```python
from build123d import *

# Parameters (mm, degrees)
F1_DEPTH = 25.4


with BuildPart() as f1:
    # F0 (on Front) → F1 (new body)
    with BuildSketch(Plane.XZ):
        with BuildLine():
            Line((69.85, 31.75), (-69.85, 31.75))
            ThreePointArc((-69.85, 31.75), (-92.30064, 22.45064), (-101.6, 0))
            ThreePointArc((-101.6, 0), (-92.30064, -22.45064), (-69.85, -31.75))
            Line((-69.85, -31.75), (69.85, -31.75))
            ThreePointArc((69.85, -31.75), (92.30064, -22.45064), (101.6, 0))
            ThreePointArc((101.6, 0), (92.30064, 22.45064), (69.85, 31.75))
        make_face()
        with BuildLine():
            Line((-69.85, 25.4), (69.85, 25.4))
            ThreePointArc((69.85, 25.4), (87.810512, 17.960512), (95.25, 0))
            ThreePointArc((95.25, 0), (87.810512, -17.960512), (69.85, -25.4))
            Line((69.85, -25.4), (-69.85, -25.4))
            ThreePointArc((-69.85, -25.4), (-87.810512, -17.960512), (-95.25, 0))
            ThreePointArc((-95.25, 0), (-87.810512, 17.960512), (-69.85, 25.4))
        make_face(mode=Mode.SUBTRACT)
    extrude(amount=F1_DEPTH)


solid = f1.part
```
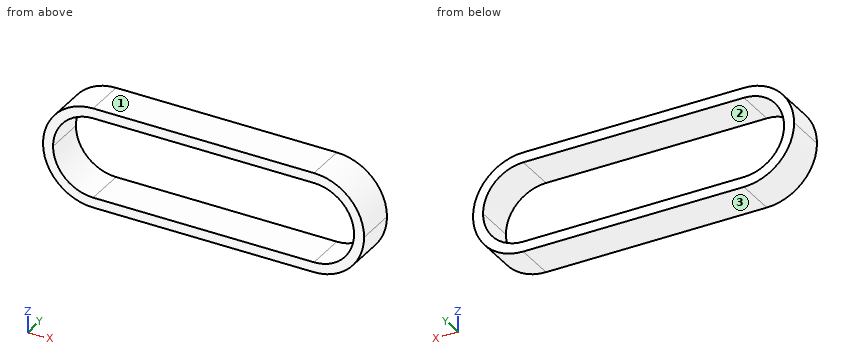
Input: part model. Units: mm. Frame: model coordinates. Face numbers are marked on the shaded views. Give positions to 0.01 mm unless a question says otherwise; leave off trailing zeros. Order: outer loops, then holes, each group sorted by start corner. A loop starts at its lowest first (then second) coordinate and runs counter-clockwise, first axis right, second up. Notation, with made-up numbers: M -17,48.5 L 25,48.5 A17 cw 25,63.5 Z; hole C 84.25,23.25 d2. An arc over 180 degrees is marked long. Return JSON: item names as keys, results as strings.
Item 1: Cut plane C-C (z = -11.5). Return loops of the section in (x, y), then the cut area to 3 significant figures.
Solutions:
{"outline": "M -99.44,-25.4 L -92.5,-25.4 L -92.5,0 L -99.44,0 Z; M 92.5,-25.4 L 99.44,-25.4 L 99.44,0 L 92.5,0 Z", "area": "353 mm^2"}
Item 2: Pull-direction query (Z, two-part tool) for the marked faces 1, 2 and 3; classes: +Z half, -Z half, draft (parallel to the pull), parting line (faces both ways), or undercut.
Solutions:
{"face 1": "+Z half", "face 2": "undercut", "face 3": "-Z half"}
Item 3: Ray query, probe 1 along Z at (x, y) = (-69, -14.25); probe 2 along X at (y, z) = (-8, -16). Return the intervals inside material, ascending.
Solutions:
{"probe 1": "-31.75 to -25.4, 25.4 to 31.75", "probe 2": "-97.27 to -89.58, 89.58 to 97.27"}
Item 4: First-contact query: P1, Ø1, axis at y = -19, z = -10, coming from the +X side; P2, Ø12, axis at x = 77, y = -21.5, coming from the -Z side; P3, Ø3, axis at y = -12.5, z = 5, coming from the -X side. Flat tips, straight axial feed; report the tip coordinate or a pass-through.
Solutions:
{"P1": "x = 100.15", "P2": "z = -31.73", "P3": "x = -101.41"}
Item 5: Cut plane A-A (x = -62). Return loops of the section in (y, z).
Solutions:
{"outline": "M -25.4,-31.75 L 0,-31.75 L 0,-25.4 L -25.4,-25.4 Z; M -25.4,25.4 L 0,25.4 L 0,31.75 L -25.4,31.75 Z"}
Item 6: Cut plane B-B (y = -22.5). Return loops of the section in (x, z), then the cut area to 3 significant figures.
Solutions:
{"outline": "M -101.6,0 A31.75 ccw -69.85,-31.75 L 69.85,-31.75 A31.75 ccw 101.6,0 A31.75 ccw 69.85,31.75 L -69.85,31.75 A31.75 ccw Z; hole M -95.25,0 A25.4 ccw -69.85,-25.4 L 69.85,-25.4 A25.4 ccw 95.25,0 A25.4 ccw 69.85,25.4 L -69.85,25.4 A25.4 ccw Z", "area": "2,910 mm^2"}
